Here's how the part is built. I have some questions about the finished solid (model axes, mm). Face numbers are marked on the shaded views. A direction names the side the tool comes from. Coordinates: 2 decimals unless noted, no trailing zeros. Write each loop counter-clockwise with the first axis right and the second up, starting at its lowest first coordinate (ties: lowest second). Pieces come first, ordered by that corner, then holes. Notation, with made-up numbers: (35, 80) -> (88, 80) arc R24 cw to (88, 118) -> close; hole circle Ø1 at (27, 45.25). An arc over 180 degrees is marked (long way). Put each result on its own line as item: value. Start each with the question number.
Item 1: I want a section at A-A, the plane x = -4. List the corners of the cut face in (y, z) for me, then the cut area to 3 significant figures.
Item 2: I want a section at B-B, the plane x = 0. List the corners of the cut face in (y, z) for me, then the cut area to 3 significant figures.
Item 3: I want a section at D-D, the plane z = 7.5. List the corners of the cut face in (x, y) for me.
Item 4: If we mould it in two halves opening along Y, with no side actions, what happens to the marked faces 4, 5 and 6? For each: released by +Y, released by -Y, zero draft, split by the parting line, or undercut.
Item 5: On a 3-axis mill with a long thin cutter (end or side, diameter ignored), from which of +Z, -Z, +X, -X, +Y, -Y can I reach the whole of each face in a straight line? I mean the marked faces 1, 2 and 3. Say none if no direction works.
Item 6: I want a section at C-C, the plane z = -3.25. List the corners of the cut face in (x, y) for me, then the cut area to 3 significant figures.
Item 7: For pin 1 (3 mm diameter, centred on x = -3, y = 10, fed in from +Z); pin 2 (1.5 mm diameter, centred on y = 10.5, z = -1.5, fed in from +X); pin 3 (6 mm diameter, centred on y = 14, z = -2, fed in from +X), each with a flat end and sliding along its axis, tell me the tip position at first contact or that it passes through.
Item 8: I need wall thicknesses on line 1 (Y direction, x = -4, z = 2.75); line 2 (X direction, y = 21.2, z = 5); line 3 (X direction, y = 15, z = 0.5). Which ranges of each line are inside material? Lowest first, please. Write a range as [from, to].
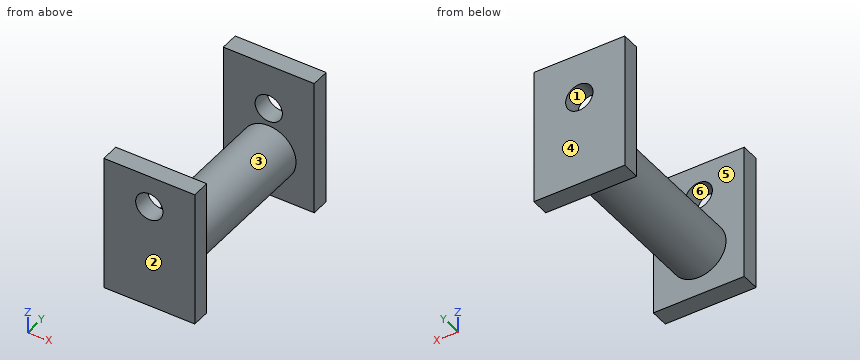
from build123d import *

# Parameters (mm, degrees)
SKETCH_1_W      = 10
SKETCH_1_H      = 15
SKETCH_1_R      = 1.5
EXTRUDE_2_DEPTH = 2
SKETCH_2_R      = 3
EXTRUDE_3_DEPTH = 20
SKETCH_3_W      = 10
SKETCH_3_H      = 15
SKETCH_3_R      = 1.5
EXTRUDE_4_DEPTH = 2


with BuildPart() as part:
    # 草图1 → 凸台-拉伸2 (new body)
    with BuildSketch(Plane(origin=(0, 0, 0), x_dir=(1, 0, 0), z_dir=(0, 1, 0))):
        with Locations((0, -2.5)):
            Rectangle(SKETCH_1_W, SKETCH_1_H)
        with Locations(Location((0, -6.5, 0), (0, 0, 270))):
            Circle(SKETCH_1_R, mode=Mode.SUBTRACT)
    extrude(amount=EXTRUDE_2_DEPTH)

    # 草图2 → 凸台-拉伸3 (add)
    with BuildSketch(Plane(origin=(0, 2, 0), x_dir=(1, 0, 0), z_dir=(0, 1, 0))):
        with Locations(Location((0, 0, 0), (0, 0, 270))):
            Circle(SKETCH_2_R)
    extrude(amount=EXTRUDE_3_DEPTH)

    # 草图3 → 凸台-拉伸4 (add)
    with BuildSketch(Plane(origin=(0, 22, 0), x_dir=(1, 0, 0), z_dir=(0, 1, 0))):
        with Locations((0, -2.5)):
            Rectangle(SKETCH_3_W, SKETCH_3_H)
        with Locations(Location((0, -5, 0), (0, 0, 270))):
            Circle(SKETCH_3_R, mode=Mode.SUBTRACT)
    extrude(amount=-EXTRUDE_4_DEPTH)


solid = part.part
Calculated:
1. outline: (0, -5) -> (2, -5) -> (2, 10) -> (0, 10) -> close; (20, -5) -> (22, -5) -> (22, 10) -> (20, 10) -> close
1. area: 60.0 mm2
2. outline: (0, -5) -> (2, -5) -> (2, -3) -> (20, -3) -> (20, -5) -> (22, -5) -> (22, 3.5) -> (20, 3.5) -> (20, 3) -> (2, 3) -> (2, 5) -> (0, 5) -> close; (0, 8) -> (2, 8) -> (2, 10) -> (0, 10) -> close; (20, 6.5) -> (22, 6.5) -> (22, 10) -> (20, 10) -> close
2. area: 156 mm2
3. outline: (-5, 0) -> (-1.12, 0) -> (-1.12, 2) -> (-5, 2) -> close; (-5, 20) -> (5, 20) -> (5, 22) -> (-5, 22) -> close; (1.12, 0) -> (5, 0) -> (5, 2) -> (1.12, 2) -> close
4. face 4: released by +Y
4. face 5: undercut
4. face 6: zero draft
5. face 1: +Y
5. face 2: +Z, -Z, +X, -X, -Y
5. face 3: none
6. outline: (-5, 0) -> (5, 0) -> (5, 2) -> (-5, 2) -> close; (-5, 20) -> (5, 20) -> (5, 22) -> (-5, 22) -> close
6. area: 40.0 mm2
7. pin 1: stops at z = 2.6
7. pin 2: stops at x = 2.9
7. pin 3: stops at x = 3
8. line 1: y = [0, 2], [20, 22]
8. line 2: x = [-5, -1.5], [1.5, 5]
8. line 3: x = [-2.96, 2.96]
